The drawing under review shows one solid part. Ordinate dimensions are in mm from its lowest x, y, z. Give positions to 0.01 mm unless a question says otherwise; leave off trailing zeros. Write each loop counter-clockwise with the first axis right and the second up, starting at its lowest first coordinate (ties: lowest second). Pieces come first, ordered by that corner, then holes. Notation, with made-up numbers: (32.25, 68) - (72.25, 68) arc R6 ccw to (72.25, 76) - close; hole circle Ø8 at (43.25, 12.25). An arc over 180 degrees is marked (long way). Write item = value, one per line.
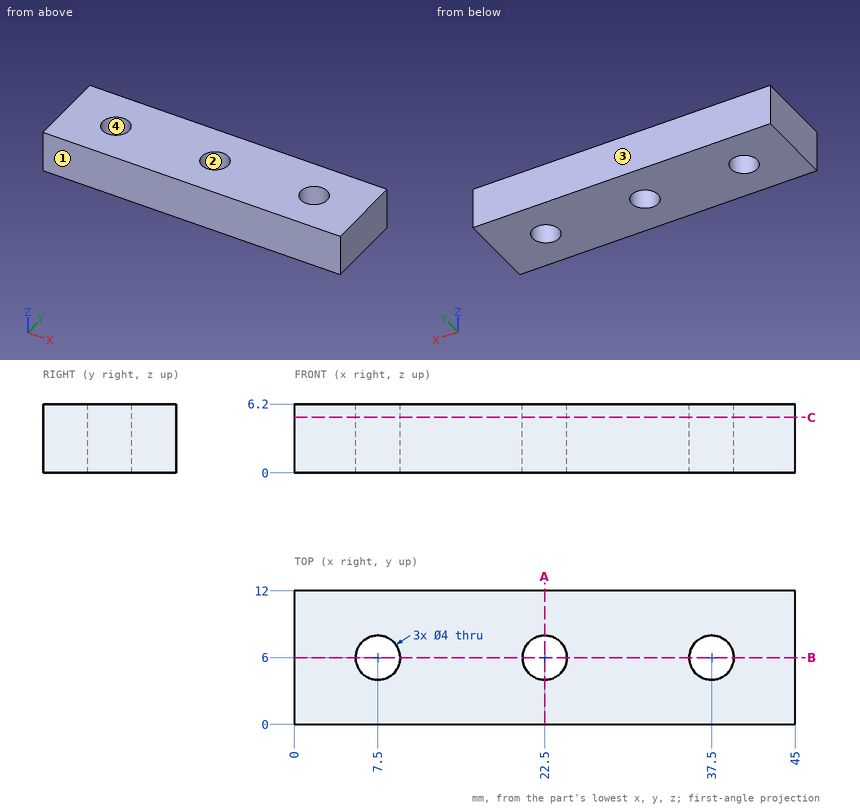
1. Take a section at A-A on x = 22.5. Give the boundary of the cut face in (y, z), and give its area (3 significant figures).
Findings below:
outline = (0, 0) - (4, 0) - (4, 6.2) - (0, 6.2) - close; (8, 0) - (12, 0) - (12, 6.2) - (8, 6.2) - close
area = 49.6 mm²
2. Draft analysis for pull direction Y (two halves, no side actions). For the marked faces 1, 2, 3 and 4, state which applies: +Y half, -Y half, draft (parallel to the pull), parting line (faces both ways), or undercut.
Findings below:
face_1 = -Y half
face_2 = undercut
face_3 = +Y half
face_4 = undercut
3. For line 1 (X direction, y = 6, z = 3.25); line 2 (Y direction, x = 22.5, z = 4.75); line 3 (Y direction, x = 38.5, z = 0.75), list the stretches that pass through material, from the lowest coordinate up. Write a range as from..to.
Findings below:
line_1 = 0..5.5, 9.5..20.5, 24.5..35.5, 39.5..45
line_2 = 0..4, 8..12
line_3 = 0..4.27, 7.73..12
4. Take a section at B-B on y = 6. Give the boundary of the cut face in (x, z).
Findings below:
outline = (0, 0) - (5.5, 0) - (5.5, 6.2) - (0, 6.2) - close; (9.5, 0) - (20.5, 0) - (20.5, 6.2) - (9.5, 6.2) - close; (24.5, 0) - (35.5, 0) - (35.5, 6.2) - (24.5, 6.2) - close; (39.5, 0) - (45, 0) - (45, 6.2) - (39.5, 6.2) - close
5. Take a section at C-C on z = 5. Give the boundary of the cut face in (x, y).
Findings below:
outline = (0, 0) - (45, 0) - (45, 12) - (0, 12) - close; hole circle Ø4 at (7.5, 6); hole circle Ø4 at (22.5, 6); hole circle Ø4 at (37.5, 6)
6. Insertion check: P1, Ø3.5, axis at x = 22.5, y = 6, coming from the +Z side; P2, Ø2, axis at x = 15.5, y = 2, coming from the -Z side. Each pin has a flat end and moves straight along its axis. Give the tip position at first contact, or say it passes through.
Findings below:
P1 = through
P2 = 0
